from build123d import *

# Parameters (mm, degrees)
BOSS_EXTRUDE1_DEPTH         = 4.7625
F_3_4_0_75_DIAMETER_HOLE1_D = 19.05
F_6_CLEARANCE_HOLE1_D       = 4.3053


with BuildPart() as part:
    # Sketch1 → Boss-Extrude1 (new body)
    with BuildSketch(Plane.XY):
        with BuildLine():
            Line((93.599, -41.275), (76.2, -41.275))
            ThreePointArc((76.2, -41.275), (64.974679849, -36.625320151), (60.325, -25.4))
            Line((60.325, -25.4), (60.325, -3.175))
            Line((60.325, -3.175), (3.175, -3.175))
            Line((3.175, -3.175), (3.175, -53.975))
            Line((3.175, -53.975), (93.599, -53.975))
            Line((93.599, -53.975), (93.599, -41.275))
        make_face()
    extrude(amount=BOSS_EXTRUDE1_DEPTH)

    # 3/4 (0.75) Diameter Hole1 (through all)
    with Locations(Plane.XY.offset(4.7625)):
        with Locations((17.526, -22.352)):
            Hole(F_3_4_0_75_DIAMETER_HOLE1_D / 2)

    # #6 Clearance Hole1 (through all)
    with Locations(Plane.XY.offset(4.7625)):
        with Locations((36.322, -16.51), (85.6615, -47.625)):
            Hole(F_6_CLEARANCE_HOLE1_D / 2)


solid = part.part
Model file for the job. Use its own axes, mm. A direction names the side the tool comes from. Give positions to 0.01 mm unless a question says otherwise; leave off trailing zeros. Loops run counter-clockwise (first coordinate to the right, second up) from the corner with the lowest first, then second, coordinate; pieces in that order, holes last.
1) Saw through at A-A (x = 9). Write the cut outline in (y, z) (1 decimal).
2) Saw through at D-D (x = 82.5). Write the cut outline in (y, z) (1 decimal), plus the area to 3 significant figures.
3) Tool access for faces 1 (the flat face through (93.599, -48, 2)), 2 (the flat face through (85, -41.275, 2)): list every direction of +Z, -Z, +X, -X, +Y, -Y with a clear straight run to the whole face (end or side of a thin tool).
4) Flat gauge pin, fed straight in: pin 1 Ø1.4 at (y, z) = (-14.5, 1.5) entering from +X (3 decimals). Where does the tip first touch, or does it go through?
5) Wall check: line 1 (X direction, y = -17, z = 4.5) (3 decimals); line 2 (Y direction, x = 22, z = 2.75) (3 decimals); line 3 (X direction, y = -49, z = 2.1) (3 decimals). Give the ranges that are in metal, low to high.
6) Pull direction X, two halves, no side cores. Call faces 3 (the flat face through (60.325, -14, 2)), 4 (the cylindrical face through (83.6, -47, 2.3)), 5 (the cylindrical face through (18.77, -12.91, 2.35)), 6 (the flat face through (38, -28, 0)): +X half, -X half, draft (parallel to the pull), parting line (faces both ways), or undercut.
7) Saw through at B-B (y = -16.51). Write the cut outline in (x, z) (1 decimal).
8) Saw through at C-C (z = 2.55). Count the separate pieces of the cut face and the enclosed holes in it, plus the area to 3 significant figures.
Answer block:
1. outline: (-54, 0) - (-26.6, 0) - (-26.6, 4.8) - (-54, 4.8) - close; (-18.1, 0) - (-3.2, 0) - (-3.2, 4.8) - (-18.1, 4.8) - close
2. outline: (-54, 0) - (-41.3, 0) - (-41.3, 4.8) - (-54, 4.8) - close
2. area: 60.5 mm2
3. face 1: +Z, -Z, +X, +Y, -Y
3. face 2: +Z, -Z, +X, +Y
4. pin 1: stops at x = 60.325
5. line 1: x = 3.175 to 9.647, 25.405 to 34.226, 38.418 to 60.325
5. line 2: y = -53.975 to -30.761, -13.943 to -3.175
5. line 3: x = 3.175 to 84.005, 87.318 to 93.599
6. face 3: +X half
6. face 4: undercut
6. face 5: undercut
6. face 6: draft
7. outline: (3.2, 0) - (10, 0) - (10, 4.8) - (3.2, 4.8) - close; (25, 0) - (34.2, 0) - (34.2, 4.8) - (25, 4.8) - close; (38.5, 0) - (60.3, 0) - (60.3, 4.8) - (38.5, 4.8) - close
8. separate pieces: 1
8. enclosed holes: 3
8. area: 3,070 mm2
